Can you work these out from the drawing? Everything is in mm from the part's minimum corner. A direction names the side the tool comes from. Coordinates: 2 decimals unless noted, no trailing zeros. Loops run counter-clockwise (first coordinate to the right, second up) from the corner with the lowest first, then second, coordinate; pieces in that order, holes last. Notation, with made-up numbers: (6, 19.25) - (46, 19.25) arc R16 cw to (46, 28.25) - close; hole circle Ø4 at (12.5, 34.25). An arc over 180 degrees is marked (long way). One line per question, with ' | ' between items. Start each with the question number.
1. I want a section at A-A, the plane z = 4.25. Write out the boundary of the cut face in (x, y), then the cut area to 3 significant figures.
2. I want a section at B-B, the plane x = 17.5. Write out the boundary of the cut face in (y, z).
3. Please list where these lines run through material, in increasing order: L1, parallel to X at y = 4, z = 7; L2, parallel to Z at x = 9, y = 26. Write a range as [from, to].
4. Which directions (+Z, -Z, +X, -X, +Y, -Y) give clear straight access to the entire face, cutting with the end or side of a thin tool? Please do the marked faces 1 and 2.
5. I'm going to push a flat-ended pin straight in: P1, Ø2, axis at x = 6.5, y = 12.5, coming from the +Z side. Where does the tip first touch, or does it pass through?
6. We'd pull the mould along X, two halves only. Please class the marked faces 3, 4, 5 and 6: pulls with the +X half, pulls with the -X half, needs draft (parallel to the pull), parting line crosses it, or undercut.
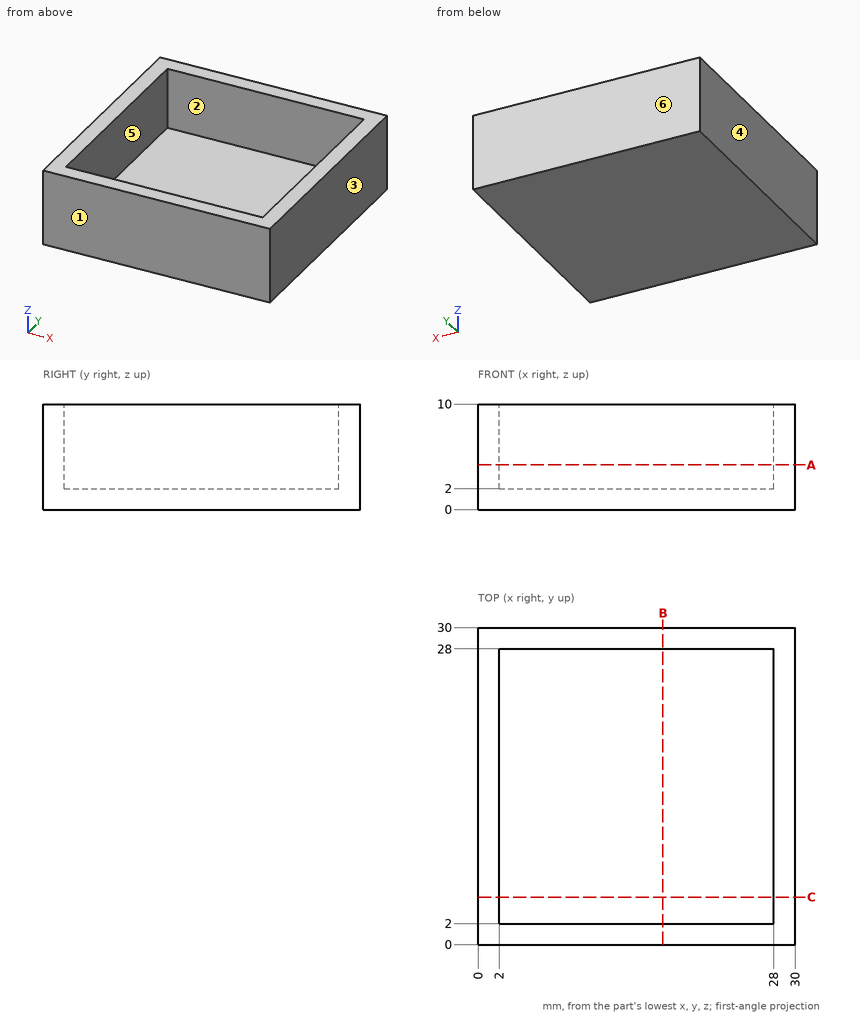
Results are:
1) outline: (0, 0) - (30, 0) - (30, 30) - (0, 30) - close; hole (2, 2) - (28, 2) - (28, 28) - (2, 28) - close | area: 224 mm2
2) outline: (0, 0) - (30, 0) - (30, 10) - (28, 10) - (28, 2) - (2, 2) - (2, 10) - (0, 10) - close
3) L1: x = [0, 2], [28, 30] | L2: z = [0, 2]
4) face 1: +Z, -Z, +X, -X, -Y | face 2: +Z
5) P1: stops at z = 2
6) face 3: pulls with the +X half | face 4: pulls with the -X half | face 5: undercut | face 6: needs draft
